Autodesk Inventor part; units mm, degrees
ref_plane "YZ Plane" through (0, 0, 0) normal (1, 0, 0) x (0, 1, 0)
ref_plane "XZ Plane" through (0, 0, 0) normal (0, 1, 0) x (-1, 0, 0)
ref_plane "XY Plane" through (0, 0, 0) normal (0, 0, 1) x (1, 0, 0)
sketch "Sketch1" plane through (0, 0, 0) normal (0, 1, 0) x (-1, 0, 0)
  line L0 (-37.2265, 95.5) -> (37.2265, 95.5)
  line L1 (37.2265, -95.5) -> (-37.2265, -95.5)
  line L2 (43, -85.5) -> (111, -85.5)
  line L3 (111, -85.5) -> (111, 85.5)
  line L4 (111, 85.5) -> (43, 85.5)
  line L5 (-37.2265, 95.5) -> (-43, 85.5)
  line L6 (-43, 85.5) -> (-43, -85.5)
  line L7 (-43, -85.5) -> (-37.2265, -95.5)
  line L8 (37.2265, -95.5) -> (43, -85.5)
  line L9 (37.2265, 95.5) -> (43, 85.5)
  point P0 (0, 0)
  point P1 (0, 0)
  point P2 (111, 0)
  dimension "d5" = 191
  dimension "d6" = 171
  dimension "d8" = 154
  dimension "d10" = 120
  dimension "d11" = 86
extrude "Extrusion1" add sketch "Sketch1" along normal mid plane 2.6
properties part number "PlayerLeaderslMats_All" material "Paper"
Here's how the part is built. I have some questions about the finished solid (model axes, mm). Coordinates: 2 decimals unless noted, no trailing zeros. Write each loop counter-clockwise with the first axis right and the second up, starting at its lowest first coordinate (ties: lowest second). Pieces come first, ordered by that corner, then holes. Notation, with made-up numbers: (89, 6.5) - (98, 6.5) arc R26 cw to (98, 36.5) - close; hole circle Ø5 at (37.25, 62). An arc over 180 degrees is marked (long way). Use one line per item in the form item = value.
1) Suppose I cut it at B-B, the plane x = -65.5. Write out the boundary of the cut face in (y, z).
Solved:
outline = (-1.3, -85.5) - (1.3, -85.5) - (1.3, 85.5) - (-1.3, 85.5) - close
2) Suppose I cut it at A-A, the plane y = 0.1. Write out the boundary of the cut face in (x, z).
Solved:
outline = (-111, -85.5) - (-43, -85.5) - (-37.23, -95.5) - (37.23, -95.5) - (43, -85.5) - (43, 85.5) - (37.23, 95.5) - (-37.23, 95.5) - (-43, 85.5) - (-111, 85.5) - close
3) I need wall thicknesses on line 1 (Z direction, x = -59.5, y = -0.25); line 2 (X direction, y = -0.8, z = 86.5). Which ranges of each line are inside material? Lowest first, please.
Solved:
line_1 = -85.5 to 85.5
line_2 = -42.42 to 42.42
4) I'm going to push flat-ended pins straight in: P1, Ø0.8, axis at x = -83, y = 0, coming from the -Z side; P2, Ø1.3, axis at x = -71, y = -0.5, coming from the +Z side. Where does each tip first touch, or does it pass through?
Solved:
P1 = -85.5
P2 = 85.5
